Geometry: final body of the model. Coordinates: model frame, mm. A direction names the side the tool comes from. Coordinates: 2 decimals unless noted, no trailing zeros. Write each loop counter-clockwise with the first axis right and the second up, starting at its lowest first coordinate (ties: lowest second). Pieces come first, ordered by that corner, then holes. Notation, with made-up numbers: M -40,70 L 15,70 A24 cw 15,82 Z; hole C 60.5,-34.5 d4. An arc over 180 degrees is marked long. Write item = value, one per line. Start each with the question number.
Item 1: Reachability of faces 1 (the flat face through (233.698, -6.261, 80.627)), 2 (the cylindrical face through (199.24, -6.26, 176.81)) from +Z, -Z, +X, -X, +Y, -Y: full face, straight path, thin tool, end or side. Return the list, or none.
Item 2: Section C-C on x = 328.5. Output: boundary loops of the cut face in (y, z).
Item 3: Pull-direction query (Z, two-part tool) for faces 3 (the flat face through (63.5, -6, 19)), 4 (the flat face through (44, -6, 25.4)), 5 (the cylindrical face through (375.96, -6.26, 192.99)), 6 (the cylindrical face through (31.736, -6.261, 47.231)); classes: +Z half, -Z half, draft (parallel to the pull), parting line (faces both ways), or undercut.
Item 4: Section B-B on x = 252. Output: boundary loops of the cut face in (y, z), plus the area to 3 significant figures.
Item 5: First-contact query: pin 1 Ø1 at (y, z) = (-11, 84) entering from +X (3 decimals); pin 2 Ø4 at (x, y) = (47.5, -8.5) entering from -Z; pin 3 Ø4 at (y, z) = (-5.5, 167.5) entering from -X. Flat tips, straight axial feed; report the tip coordinate or a pass-through.
Item 6: Ray query, L1, parallel to Z at x = 228.5, y = -2.25; L2, parallel to Z at x = 381, y = -7.75; L3, parallel to Z at x = 330, y = -2. Return the intervals inside material, ascending. Write a range as [from, to].
from build123d import *

# Parameters (mm, degrees)
F0_R     = 6.35
F1_DEPTH = 12.7


with BuildPart() as f1:
    # F0 (on Front) → F1 (new body)
    with BuildSketch(Plane.XZ):
        with BuildLine():
            ThreePointArc((44.034086, 65.603644), (31.603262, 46.945036), (25.4, 25.4))
            Line((25.4, 25.4), (63.5, 25.4))
            Line((63.5, 25.4), (63.5, 12.7))
            ThreePointArc((63.5, 12.7), (154.429017, 34.504579), (238.125, 76.2))
            Line((238.125, 76.2), (229.144744, 85.180256))
            ThreePointArc((229.144744, 85.180256), (223.299522, 101.436404), (232.111116, 116.295232))
            ThreePointArc((232.111116, 116.295232), (304.972177, 155.20276), (384.335327, 178.094252))
            ThreePointArc((384.335327, 178.094252), (362.032394, 195.08013), (380.807759, 215.89903))
            ThreePointArc((380.807759, 215.89903), (196.809301, 175.733004), (44.034086, 65.603644))
        make_face()
        with BuildLine():
            ThreePointArc((400.05, 196.85), (394.402244, 210.388181), (380.807759, 215.89903))
            ThreePointArc((380.807759, 215.89903), (362.032394, 195.08013), (384.335327, 178.094252))
            ThreePointArc((384.335327, 178.094252), (395.602063, 184.61553), (400.05, 196.85))
        make_face()
        with Locations((381, 196.85)):
            Circle(F0_R, mode=Mode.SUBTRACT)
    extrude(amount=F1_DEPTH)


solid = f1.part
Responses:
q1.face_1 = +X, +Y, -Y
q1.face_2 = +Z, -X, +Y, -Y
q2.outline = M -12.7,163.89 L 0,163.89 L 0,212.4 L -12.7,212.4 Z
q3.face_3 = draft
q3.face_4 = -Z half
q3.face_5 = undercut
q3.face_6 = +Z half
q4.outline = M -12.7,128.92 L 0,128.92 L 0,196.26 L -12.7,196.26 Z
q4.area = 855 mm²
q5.pin_1 = 230.825
q5.pin_2 = 25.4
q5.pin_3 = 175.37
q6.L1 = [70.14, 85.86], [113.17, 188.5]
q6.L2 = [177.49, 190.5], [203.2, 215.9]
q6.L3 = [164.39, 212.59]
